```python
from build123d import *

# Parameters (mm, degrees)
SKETCH1_R           = 2.75
BOSS_EXTRUDE1_DEPTH = 5
CHAMFER1_SIZE       = 1
SKETCH2_R           = 1.5
CUT_EXTRUDE1_DEPTH  = 83.773788122
BOSS_EXTRUDE2_START = 5
SKETCH3_W           = 5.5
SKETCH3_H           = 5.5
SKETCH3_W_2         = 3
SKETCH3_H_2         = 3
BOSS_EXTRUDE2_DEPTH = 5
CHAMFER3_SIZE       = 0.5


with BuildPart() as part:
    # Sketch1 → Boss-Extrude1 (new body)
    with BuildSketch(Plane.XY):
        Polygon((82.5, 4.5), (82.5, -4.5), (0, -4.5), (-19, -2.75), (-19, 2.75), (0, 4.5), align=None)
        Circle(SKETCH1_R, mode=Mode.SUBTRACT)
    extrude(amount=BOSS_EXTRUDE1_DEPTH)

    # Chamfer1
    # the kernel refuses this chamfer: 1 mm, written as the material it takes off along each edge
    with BuildSketch(Plane(origin=(-12.85841494, 4.5, 5), x_dir=(0, 0, -1), z_dir=(1, 0, 0)), Plane(origin=(85.071682988, -4.5, 5), x_dir=(0, 0, -1), z_dir=(-1, 0, 0))) as chamfer1_piece_1:
        Polygon((CHAMFER1_SIZE, 0), (0, -CHAMFER1_SIZE), (0, 0), align=None)
    extrude(amount=97.930097928, mode=Mode.SUBTRACT)
    with BuildSketch(Plane(origin=(-12.85841494, 4.5, 0), x_dir=(0, 0, 1), z_dir=(1, 0, 0)), Plane(origin=(85.071682988, -4.5, 0), x_dir=(0, 0, 1), z_dir=(-1, 0, 0))) as chamfer1_piece_2:
        Polygon((CHAMFER1_SIZE, 0), (0, CHAMFER1_SIZE), (0, 0), align=None)
    extrude(amount=97.930097928, mode=Mode.SUBTRACT)

    # Sketch2 → Cut-Extrude1 (cut, through all)
    with BuildSketch(Plane.XY.offset(5)):
        with Locations((-14, 0)):
            Circle(SKETCH2_R)
    extrude(amount=-CUT_EXTRUDE1_DEPTH, mode=Mode.SUBTRACT)

    # Sketch3 → Boss-Extrude2 (add)
    # profile 1 of 5: a face of its own
    with BuildSketch(Plane.XY.offset(5).offset(BOSS_EXTRUDE2_START)):
        with Locations((-14, 0)):
            Rectangle(SKETCH3_W, SKETCH3_H)
        with Locations((-14, 0)):
            Rectangle(SKETCH3_W_2, SKETCH3_H_2, mode=Mode.SUBTRACT)
    # profile 2 of 5: a face of its own
    with BuildSketch(Plane.XY.offset(5).offset(BOSS_EXTRUDE2_START)):
        with BuildLine():
            Line((-15.5, 1.5), (-15.5, 3e-09))
            ThreePointArc((-15.5, 3e-09), (-15.060660171, 1.060660173), (-14, 1.5))
            Line((-14, 1.5), (-15.5, 1.5))
        make_face()
    # profile 3 of 5: a face of its own
    with BuildSketch(Plane.XY.offset(5).offset(BOSS_EXTRUDE2_START)):
        with BuildLine():
            Line((-15.5, 3e-09), (-15.5, -1.5))
            Line((-15.5, -1.5), (-14, -1.5))
            ThreePointArc((-14, -1.5), (-15.060660173, -1.060660171), (-15.5, 3e-09))
        make_face()
    # profile 4 of 5: a face of its own
    with BuildSketch(Plane.XY.offset(5).offset(BOSS_EXTRUDE2_START)):
        with BuildLine():
            ThreePointArc((-12.5, 0), (-12.939339828, -1.060660172), (-14, -1.5))
            Line((-14, -1.5), (-12.5, -1.5))
            Line((-12.5, -1.5), (-12.5, 0))
        make_face()
    # profile 5 of 5: a face of its own
    with BuildSketch(Plane.XY.offset(5).offset(BOSS_EXTRUDE2_START)):
        with BuildLine():
            ThreePointArc((-14, 1.5), (-12.939339828, 1.060660172), (-12.5, 0))
            Line((-12.5, 0), (-12.5, 1.5))
            Line((-12.5, 1.5), (-14, 1.5))
        make_face()
    extrude(amount=-BOSS_EXTRUDE2_DEPTH)

    # Chamfer3
    # the kernel refuses this chamfer: 0.5 mm, written as the material it adds along each edge
    with BuildSketch(Plane(origin=(-16.75, -2.75, 5), x_dir=(0, -1, 0), z_dir=(1, 0, 0))) as chamfer3_piece_1_section:
        Polygon((CHAMFER3_SIZE, 0), (0, -CHAMFER3_SIZE), (0, 0), align=None)
    chamfer3_piece_1 = extrude(amount=5.5, mode=Mode.PRIVATE)
    chamfer3_piece_1 = split(chamfer3_piece_1, bisect_by=Plane(origin=(-16.768927039, -2.955493562, 5), z_dir=(0.09171704949125846, 0.995785108762236, 0)), keep=Keep.TOP, mode=Mode.PRIVATE)
    add(chamfer3_piece_1)
    with BuildSketch(Plane(origin=(-11.25, -2.75, 5), x_dir=(1, 0, 0), z_dir=(0, 1, 0)), Plane(origin=(-16.75, 2.75, 5), x_dir=(-1, 0, 0), z_dir=(0, -1, 0))) as chamfer3_piece_2:
        Polygon((CHAMFER3_SIZE, 0), (0, -CHAMFER3_SIZE), (0, 0), align=None)
    extrude(amount=5.5)
    with BuildSketch(Plane(origin=(-11.25, 2.75, 5), x_dir=(0, 1, 0), z_dir=(-1, 0, 0))) as chamfer3_piece_3_section:
        Polygon((CHAMFER3_SIZE, 0), (0, -CHAMFER3_SIZE), (0, 0), align=None)
    chamfer3_piece_3 = extrude(amount=5.5, mode=Mode.PRIVATE)
    chamfer3_piece_3 = split(chamfer3_piece_3, bisect_by=Plane(origin=(-11.315193133, 3.457811159, 5), z_dir=(0.09171704949125607, -0.9957851087622361, 0)), keep=Keep.TOP, mode=Mode.PRIVATE)
    add(chamfer3_piece_3)
    with BuildSketch(Plane(origin=(-16.75, 2.75, 5), x_dir=(-1, 0, 0), z_dir=(0, -1, 0))) as chamfer3_piece_4a_section:
        Polygon((CHAMFER3_SIZE, 0), (0, -CHAMFER3_SIZE), (0, 0), align=None)
    chamfer3_piece_4a = extrude(amount=6.785841494, mode=Mode.PRIVATE)
    chamfer3_piece_4a = split(chamfer3_piece_4a, bisect_by=Plane(origin=(-17.271244635, -2.909227468, 5), z_dir=(0.09171704949125846, 0.995785108762236, 0)), keep=Keep.TOP, mode=Mode.PRIVATE)
    chamfer3_piece_4a = split(chamfer3_piece_4a, bisect_by=Plane(origin=(-16.75, -2.75, 5), z_dir=(0, -1, 0)), keep=Keep.TOP, mode=Mode.PRIVATE)
    with BuildSketch(Plane(origin=(-18.035841494, -2.75, 5), x_dir=(0, -1, 0), z_dir=(1, 0, 0))) as chamfer3_piece_4b_section:
        Polygon((CHAMFER3_SIZE, 0), (0, -CHAMFER3_SIZE), (0, 0), align=None)
    chamfer3_piece_4b = extrude(amount=6.785841494, mode=Mode.PRIVATE)
    chamfer3_piece_4b = split(chamfer3_piece_4b, bisect_by=Plane(origin=(-18.043952012, -2.838057052, 5), z_dir=(0.09171704949125846, 0.995785108762236, 0)), keep=Keep.TOP, mode=Mode.PRIVATE)
    chamfer3_piece_4b = split(chamfer3_piece_4b, bisect_by=Plane(origin=(-16.75, -2.75, 5), z_dir=(-1, 0, 0)), keep=Keep.TOP, mode=Mode.PRIVATE)
    chamfer3_piece_4 = chamfer3_piece_4a & chamfer3_piece_4b
    add(chamfer3_piece_4)
    with BuildSketch(Plane(origin=(-11.25, -4.035841494, 5), x_dir=(1, 0, 0), z_dir=(0, 1, 0))) as chamfer3_piece_5a_section:
        Polygon((CHAMFER3_SIZE, 0), (0, -CHAMFER3_SIZE), (0, 0), align=None)
    chamfer3_piece_5a = extrude(amount=6.785841494, mode=Mode.PRIVATE)
    chamfer3_piece_5a = split(chamfer3_piece_5a, bisect_by=Plane(origin=(-11.25, -3.767920747, 4.732079253), z_dir=(0, 0.7071067811865476, -0.7071067811865476)), keep=Keep.TOP, mode=Mode.PRIVATE)
    chamfer3_piece_5a = split(chamfer3_piece_5a, bisect_by=Plane(origin=(-11.197756622, -3.46862768, 5), z_dir=(0.09171704949125846, 0.995785108762236, 0)), keep=Keep.TOP, mode=Mode.PRIVATE)
    chamfer3_piece_5a = split(chamfer3_piece_5a, bisect_by=Plane(origin=(-11.25, -2.75, 5), z_dir=(0, -1, 0)), keep=Keep.TOP, mode=Mode.PRIVATE)
    with BuildSketch(Plane(origin=(-16.75, -2.75, 5), x_dir=(0, -1, 0), z_dir=(1, 0, 0))) as chamfer3_piece_5b_section:
        Polygon((CHAMFER3_SIZE, 0), (0, -CHAMFER3_SIZE), (0, 0), align=None)
    chamfer3_piece_5b = extrude(amount=6.785841494, mode=Mode.PRIVATE)
    chamfer3_piece_5b = split(chamfer3_piece_5b, bisect_by=Plane(origin=(-11.25, -2.75, 5), z_dir=(1, 0, 0)), keep=Keep.TOP, mode=Mode.PRIVATE)
    chamfer3_piece_5 = chamfer3_piece_5a & chamfer3_piece_5b
    add(chamfer3_piece_5)
    with BuildSketch(Plane(origin=(-9.964158506, 2.75, 5), x_dir=(0, 1, 0), z_dir=(-1, 0, 0))) as chamfer3_piece_6a_section:
        Polygon((CHAMFER3_SIZE, 0), (0, -CHAMFER3_SIZE), (0, 0), align=None)
    chamfer3_piece_6a = extrude(amount=6.785841494, mode=Mode.PRIVATE)
    chamfer3_piece_6a = split(chamfer3_piece_6a, bisect_by=Plane(origin=(-11.25, 2.75, 5), z_dir=(1, 0, 0)), keep=Keep.TOP, mode=Mode.PRIVATE)
    with BuildSketch(Plane(origin=(-11.25, -2.75, 5), x_dir=(1, 0, 0), z_dir=(0, 1, 0))) as chamfer3_piece_6b_section:
        Polygon((CHAMFER3_SIZE, 0), (0, -CHAMFER3_SIZE), (0, 0), align=None)
    chamfer3_piece_6b = extrude(amount=6.785841494, mode=Mode.PRIVATE)
    chamfer3_piece_6b = split(chamfer3_piece_6b, bisect_by=Plane(origin=(-11.25, 0.375, 8.125), z_dir=(0, -0.7071067811865476, -0.7071067811865476)), keep=Keep.TOP, mode=Mode.PRIVATE)
    chamfer3_piece_6b = split(chamfer3_piece_6b, bisect_by=Plane(origin=(-11.81751073, 3.411545064, 5), z_dir=(0.09171704949125607, -0.9957851087622361, 0)), keep=Keep.TOP, mode=Mode.PRIVATE)
    chamfer3_piece_6b = split(chamfer3_piece_6b, bisect_by=Plane(origin=(-11.25, 2.75, 5), z_dir=(0, 1, 0)), keep=Keep.TOP, mode=Mode.PRIVATE)
    chamfer3_piece_6 = chamfer3_piece_6a & chamfer3_piece_6b
    add(chamfer3_piece_6)
    with BuildSketch(Plane(origin=(-16.75, 4.035841494, 5), x_dir=(-1, 0, 0), z_dir=(0, -1, 0))) as chamfer3_piece_7a_section:
        Polygon((CHAMFER3_SIZE, 0), (0, -CHAMFER3_SIZE), (0, 0), align=None)
    chamfer3_piece_7a = extrude(amount=6.785841494, mode=Mode.PRIVATE)
    chamfer3_piece_7a = split(chamfer3_piece_7a, bisect_by=Plane(origin=(-16.651490528, 2.966310083, 5), z_dir=(0.09171704949125607, -0.9957851087622361, 0)), keep=Keep.TOP, mode=Mode.PRIVATE)
    chamfer3_piece_7a = split(chamfer3_piece_7a, bisect_by=Plane(origin=(-16.75, 2.75, 5), z_dir=(0, 1, 0)), keep=Keep.TOP, mode=Mode.PRIVATE)
    with BuildSketch(Plane(origin=(-11.25, 2.75, 5), x_dir=(0, 1, 0), z_dir=(-1, 0, 0))) as chamfer3_piece_7b_section:
        Polygon((CHAMFER3_SIZE, 0), (0, -CHAMFER3_SIZE), (0, 0), align=None)
    chamfer3_piece_7b = extrude(amount=6.785841494, mode=Mode.PRIVATE)
    chamfer3_piece_7b = split(chamfer3_piece_7b, bisect_by=Plane(origin=(-11.315193133, 3.457811159, 5), z_dir=(0.09171704949125607, -0.9957851087622361, 0)), keep=Keep.TOP, mode=Mode.PRIVATE)
    chamfer3_piece_7b = split(chamfer3_piece_7b, bisect_by=Plane(origin=(-16.75, 2.75, 5), z_dir=(-1, 0, 0)), keep=Keep.TOP, mode=Mode.PRIVATE)
    chamfer3_piece_7 = chamfer3_piece_7a & chamfer3_piece_7b
    add(chamfer3_piece_7)
    # the kernel refuses this chamfer: 0.5 mm, written as the material it takes off along each edge
    with BuildSketch(Plane(origin=(-9.964158506, 2.75, 10), x_dir=(0, 0, -1), z_dir=(-1, 0, 0)), Plane(origin=(-18.035841494, -2.75, 10), x_dir=(0, 0, -1), z_dir=(1, 0, 0)), Plane(origin=(-11.25, -4.035841494, 10), x_dir=(0, 0, -1), z_dir=(0, 1, 0))) as chamfer3_2_piece_1:
        Polygon((CHAMFER3_SIZE, 0), (0, CHAMFER3_SIZE), (0, 0), align=None)
    extrude(amount=8.071682988, mode=Mode.SUBTRACT)
    with BuildSketch(Plane(origin=(-16.75, 4.035841494, 10), x_dir=(1, 0, 0), z_dir=(0, -1, 0))) as chamfer3_2_piece_2:
        Polygon((CHAMFER3_SIZE, 0), (0, -CHAMFER3_SIZE), (0, 0), align=None)
    extrude(amount=8.071682988, mode=Mode.SUBTRACT)


solid = part.part
```
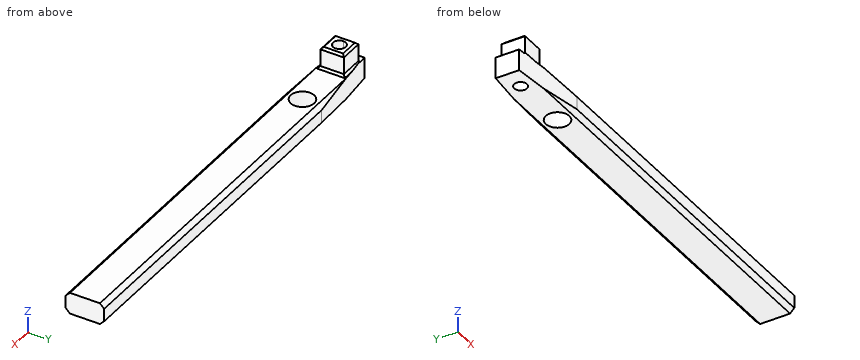
Work out the finished part from the listing and answer in its coordinate system (mm). Give positions to 0.01 mm unless a question says otherwise; leave off trailing zeros. Loops run counter-clockwise (first coordinate to the right, second up) from the corner with the lowest first, then second, coordinate; pieces in that order, holes last. Notation, with made-up numbers: (25, 38) -> (59, 38) arc R18 cw to (59, 52) -> close; hole circle Ø10 at (-2, 78). An arc over 180 degrees is marked (long way). Write item = value, one per line. Start each with the question number.
(1) Given pin 1 Ø1.2 at (y, z) = (-1, 7.5) entering from -X; pin 2 Ø1.9 at (x, y) = (-18, -0.5) entering from +Z; pin 3 Ø1.2 at (x, z) = (-14, 8) entering from +Y; pin 4 Ø6 at (x, z) = (7.5, 8.5) entering from +Y, each flat-ended and moving along its own axis, determine where each tip first touches the part or whether it passes through.
(2) Find section C-C on x = 41.5. Give the vertices of the cut face in (y, z), and give its area (3 significant figures).
(3) Find section D-D on x = -9.5. Give the vertices of the cut face in (y, z) (3 decimals), and give its area (3 significant figures).
(4) Find section B-B on z = 2.5. Give the vertices of the cut face in (x, y).
(5) Find the intervals of material crossed by probe 1 along Y at (x, z) = (0, 3.55); probe 2 along Z at (x, y) = (-1, 2.75); probe 3 along Y at (x, z) = (-14, 1.65), in increasing order. Write a range as from..to.
(6) Find section A-A on z = 6.5. Give the vertices of the cut face in (x, y).
From the geometry:
q1.pin_1 = -16.75
q1.pin_2 = 5.2
q1.pin_3 = 2.75
q1.pin_4 = through
q2.outline = (-4.5, 1) -> (-3.5, 0) -> (3.5, 0) -> (4.5, 1) -> (4.5, 4) -> (3.5, 5) -> (-3.5, 5) -> (-4.5, 4) -> close
q2.area = 43.0 mm^2
q3.outline = (-3.625, 0.125) -> (-3.5, 0) -> (3.5, 0) -> (3.625, 0.125) -> (3.625, 4.875) -> (3.5, 5) -> (-3.5, 5) -> (-3.625, 4.875) -> close
q3.area = 36.2 mm^2
q4.outline = (-19, -2.75) -> (0, -4.5) -> (82.5, -4.5) -> (82.5, 4.5) -> (0, 4.5) -> (-19, 2.75) -> close; hole circle Ø3 at (-14, 0); hole circle Ø5.5 at (0, 0)
q5.probe_1 = -4.5..-2.75, 2.75..4.5
q5.probe_2 = 0..5
q5.probe_3 = -3.21..-1.5, 1.5..3.21
q6.outline = (-16.75, -2.75) -> (-11.25, -2.75) -> (-11.25, 2.75) -> (-16.75, 2.75) -> close; hole circle Ø3 at (-14, 0)
